For this review, take the finished solid that the model builds, in its own axes (mm). A direction names the side the tool comes from. Round coordinates to 2 decimals unless told otherwise and drop trailing zeros. Order: outer loops, then holes, each group sorted by start corner. A loop starts at its lowest first (then second) coordinate and runs counter-clockwise, first axis right, second up. Notation, with made-up numbers: (-18, 77) -> (31, 77) arc R21 ccw to (31, 99) -> close; hole circle Ø4 at (54, -30). An arc over 180 degrees is marked (long way). Put each result on its own line as item: value. Start each with the question number.
```python
from build123d import *

# Parameters (mm, degrees)
F0_W     = 120
F0_H     = 120
F0_R     = 57
F1_DEPTH = 25
F2_W     = 115
F2_H     = 115
F2_R     = 22.5
F3_DEPTH = 2
F2_R_2   = 20
F4_DEPTH = 110
F5_R     = 22.5
F5_R_2   = 20
F6_DEPTH = 2


with BuildPart() as f1:
    # F0 (on Top) → F1 (new body)
    with BuildSketch(Plane.XY):
        Rectangle(F0_W, F0_H)
        Circle(F0_R, mode=Mode.SUBTRACT)
    extrude(amount=-F1_DEPTH)

    # F2 (on Top) → F3 (join)
    with BuildSketch(Plane.XY):
        Rectangle(F2_W, F2_H)
        with Locations((-32.354934313, 0)):
            Circle(F2_R, mode=Mode.SUBTRACT)
        with Locations((32.645065687, 0)):
            Circle(F2_R, mode=Mode.SUBTRACT)
    extrude(amount=F3_DEPTH)

    # F2 (on Top) → F4 (join)
    with BuildSketch(Plane.XY):
        with Locations((-32.354934313, 0)):
            Circle(F2_R)
        with Locations((-32.354934313, 0)):
            Circle(F2_R_2, mode=Mode.SUBTRACT)
        with Locations((32.645065687, 0)):
            Circle(F2_R)
        with Locations((32.645065687, 0)):
            Circle(F2_R_2, mode=Mode.SUBTRACT)
    extrude(amount=F4_DEPTH)

    # F5 (on face) → F6 (join)
    with BuildSketch(Plane.XY.offset(110)):
        with Locations((32.645065687, 0)):
            Circle(F5_R)
        with Locations((32.645065687, 0)):
            Circle(F5_R_2, mode=Mode.SUBTRACT)
        with Locations((-32.2491377592, 0)):
            Circle(F5_R)
        with Locations((32.645065687, 0)):
            Circle(F5_R_2)
    extrude(amount=F6_DEPTH)


solid = f1.part
```
Item 1: Insertion check: pin 1 Ø3 at (x, y) = (29, 11) entering from -Z; pin 2 Ø12 at (x, y) = (-8.5, 39.5) entering from +Z; pin 3 Ø1.6 at (y, z) = (-19.5, 0.5) entering from +X; pin 4 Ø12 at (y, z) = (-2, 71.5) entering from -X. Each pin has a flat end and moves straight along its axis. Give the tip position at first contact, or say it passes through.
Item 2: Mouldability with a two-part tool opening along X and no side actions: class faces 4 (the face through (60, -1, -12)), 5 (the face through (-52.336, 0.879, 54.23)), 6 (the face through (32, 0, 112)) as +X half, -X half, draft (parallel to the pull), parting line (faces both ways), or undercut.
Item 3: For L1, parallel to X at y = -9, z = 95.5; L2, parallel to X at y = -13, z = 27; L3, parallel to Y at x = 0, z = -6, list the stretches that pass through material, from the lowest coordinate up.
Item 4: Consider section A-A, the plane z = 79.5. Write out the cut boundary in (x, y).
Item 5: Consider section C-C, the plane x = 0. Write out the cut boundary in (y, z), plus the area to 3 significant figures.
Item 6: Tool access review of faces 1 (the face through (52.654, -21.831, -12.325)), 2 (the face through (-1, -60, -12)), 3 (the face through (-21.867, -19.961, 110.986)): name each direction out of +Z, -Z, +X, -X, +Y, -Y from which nothing blocks a thin tool from reaching the whole face with its end or side.
Evaluation:
1. pin 1: stops at z = 110
1. pin 2: stops at z = 2
1. pin 3: stops at x = 60
1. pin 4: stops at x = -54.85
2. face 4: +X half
2. face 5: undercut
2. face 6: draft
3. L1: x = -52.98 to -50.22, -14.49 to -11.73, 12.02 to 14.78, 50.51 to 53.27
3. L2: x = -50.72 to -47.55, -17.16 to -13.99, 14.28 to 17.45, 47.84 to 51.01
3. L3: y = -60 to -57, 57 to 60
4. outline: circle Ø45 at (-32.35, 0); circle Ø45 at (32.65, 0); hole circle Ø40 at (-32.35, 0); hole circle Ø40 at (32.65, 0)
5. outline: (-60, -25) -> (-57, -25) -> (-57, 0) -> (57, 0) -> (57, -25) -> (60, -25) -> (60, 0) -> (57.5, 0) -> (57.5, 2) -> (-57.5, 2) -> (-57.5, 0) -> (-60, 0) -> close
5. area: 380 mm^2
6. face 1: -Z
6. face 2: +Z, -Z, +X, -X, -Y
6. face 3: +Z
